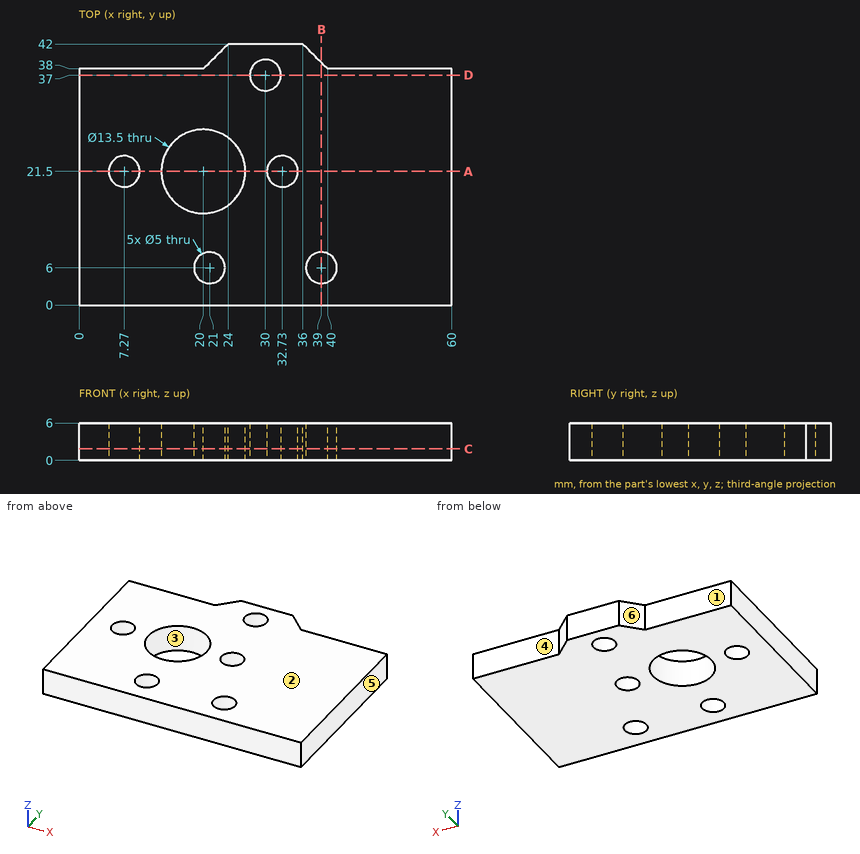
Verification items for this drawing (mm, ordinates from the low corner). A direction names the side the tool comes from. Coordinates: 2 decimals unless noted, no trailing zeros. Loops run counter-clockwise (first coordinate to the right, second up) from the corner with the lowest first, then second, coordinate; pieces in that order, holes last.
Item 1: Release check for a two-part mould opening along X. For the marked faces 3, 4, 5 and 6 record: released by +X, released by -X, zero draft, split by the parting line, or undercut.
Item 2: Sectioned sample at C-C, the plane z = 1.85. Record the boundary of the cut face in (x, y), then the cut area to 3 significant figures.
Item 3: Sectioned sample at D-D, the plane y = 37. Record the boundary of the cut face in (x, z), then the cut area to 3 significant figures.
Item 4: Thickness scan on line 1 (X direction, y = 5, z = 1.25); line 2 (Y direction, x = 32.73, z = 1.3); line 3 (Y direction, x = 7.27, z = 3.45). Record the ranges inside material, lowest first.
Item 5: Sectioned sample at A-A, the plane y = 21.5. Record the boundary of the cut face in (x, z), then the cut area to 3 significant figures.
Item 6: Go/stop test with flat-tipped pins: pin 1 Ø6.5 at (x, y) = (39, 6) entering from -Z; pin 2 Ø3 at (x, z) = (14, 2) entering from +Y. Record where each tip stops, or that it passes through.
Item 7: Access from +Z, -Z, +X, -X, +Y, -Y to the whole of each face (thin tool, end or side, straight path). Record for the marked faces 1 and 2.
Item 8: Sectioned sample at B-B, the plane x = 39. Record the boundary of the cut face in (y, z).
Check result:
1. face 3: undercut
1. face 4: zero draft
1. face 5: released by +X
1. face 6: released by -X
2. outline: (0, 0) - (60, 0) - (60, 38) - (40, 38) - (36, 42) - (24, 42) - (20, 38) - (0, 38) - close; hole circle Ø5 at (7.27, 21.5); hole circle Ø13.5 at (20, 21.5); hole circle Ø5 at (21, 6); hole circle Ø5 at (30, 37); hole circle Ø5 at (32.73, 21.5); hole circle Ø5 at (39, 6)
2. area: 2,100 mm2
3. outline: (0, 0) - (27.5, 0) - (27.5, 6) - (0, 6) - close; (32.5, 0) - (60, 0) - (60, 6) - (32.5, 6) - close
3. area: 330 mm2
4. line 1: x = 0 to 18.71, 23.29 to 36.71, 41.29 to 60
4. line 2: y = 0 to 19, 24 to 42
4. line 3: y = 0 to 19, 24 to 38
5. outline: (0, 0) - (4.77, 0) - (4.77, 6) - (0, 6) - close; (9.77, 0) - (13.25, 0) - (13.25, 6) - (9.77, 6) - close; (26.75, 0) - (30.23, 0) - (30.23, 6) - (26.75, 6) - close; (35.23, 0) - (60, 0) - (60, 6) - (35.23, 6) - close
5. area: 219 mm2
6. pin 1: stops at z = 0
6. pin 2: stops at y = 38
7. face 1: +Z, -Z, -X, +Y
7. face 2: +Z, +X, -X, +Y, -Y
8. outline: (0, 0) - (3.5, 0) - (3.5, 6) - (0, 6) - close; (8.5, 0) - (39, 0) - (39, 6) - (8.5, 6) - close
